Here's how the part is built. I have some questions about the finished solid (model axes, mm). Face numbers are marked on the shaded views. A direction names the side the tool comes from. Coordinates: 2 decimals unless noted, no trailing zeros. Loops run counter-clockwise (first coordinate to the right, second up) from the corner with the lowest first, then second, coordinate; pieces in that order, holes last. Notation, with made-up numbers: M 23.25,-1 L 33.25,-1 A29 ccw 33.25,30 Z; hole C 75.5,-5.75 d1. An arc over 180 degrees is marked long. Use one line per item in the form item = value. Start each with the question number.
(1) Imagine slicing it at C-C, the plane y = 4.75. Please give me the cut outline in (x, z).
(2) Imagine slicing it at D-D, the plane z = 0. Please give me the cut outline in (x, y).
(3) Imagine slicing it at B-B, the plane z = 7.25. Please give me the cut outline in (x, y), and give its area (3 significant figures).
(4) On a 3-axis mill with a long thin cutter (end or side, diameter ignored), from which of +Z, -Z, +X, -X, +Y, -Y can I reach the whole of each face in a straight line? I mean the marked faces 5, 6, 7 and 8. Say none if no direction works.
(5) Please list where these lines run through material, in increasing order: L1, parallel to Z at x = 11.5, y = 3.25; L2, parallel to Z at x = 0, y = 7; L3, parallel to X at y = 6.5, z = 0.
(6) Thinking about a two-plate mould opening in X: for the marked faces 1, 2, 3 and 4, which applies, +X half, -X half, draft (parallel to the pull), parting line (faces both ways), or undercut?
(7) Will these pins go through, and if not, where does the flat tip stop? P1, Ø5, axis at x = 21, y = 5, coming from the -Z side; P2, Ø12, axis at x = -0.5, z = 2.5, coming from the +Y side; P3, Ø1, axis at x = 16, y = 1.5, coming from the +Z side.
(8) Imagine slicing it at A-A, the plane x = 32. Please give me the cut outline in (y, z), and give its area (3 significant figures).
```python
from build123d import *

# Parameters (mm, degrees)
EXTRUDE_1_DEPTH     = 10
SKETCH_2_W          = 5
SKETCH_2_H          = 10
CUT_EXTRUDE_1_DEPTH = 10


with BuildPart() as part:
    # 草图1 → 凸台-拉伸1 (new body)
    with BuildSketch(Plane(origin=(0, 0, 0), x_dir=(1, 0, 0), z_dir=(0, 1, 0))):
        with BuildLine():
            ThreePointArc((11.180339887, 10), (12.90569415, 7.644805982), (14.142135624, 5))
            Line((14.142135624, 5), (50, 5))
            Line((50, 5), (55, 5))
            Line((55, 5), (55, 10))
            Line((55, 10), (11.180339887, 10))
        make_face()
        with BuildLine():
            Line((8.947765084, 5), (14.142135624, 5))
            ThreePointArc((14.142135624, 5), (12.90569415, 7.644805982), (11.180339887, 10))
            ThreePointArc((11.180339887, 10), (-15, 0), (11.180339887, -10))
            ThreePointArc((11.180339887, -10), (12.90569415, -7.644805982), (14.142135624, -5))
            Line((14.142135624, -5), (8.947765084, -5))
            ThreePointArc((8.947765084, -5), (-10.25, 0), (8.947765084, 5))
        make_face()
        with BuildLine():
            Line((50, -5), (14.142135624, -5))
            ThreePointArc((14.142135624, -5), (12.90569415, -7.644805982), (11.180339887, -10))
            Line((11.180339887, -10), (55, -10))
            Line((55, -10), (55, -5))
            Line((55, -5), (50, -5))
        make_face()
    extrude(amount=EXTRUDE_1_DEPTH)

    # 草图2 → 切除-拉伸1 (cut)
    with BuildSketch(Plane(origin=(55, 0, 0), x_dir=(0, 0, -1), z_dir=(1, 0, 0))):
        with Locations((7.5, 5)):
            Rectangle(SKETCH_2_W, SKETCH_2_H)
        with Locations((-7.5, 5)):
            Rectangle(SKETCH_2_W, SKETCH_2_H)
    extrude(amount=-CUT_EXTRUDE_1_DEPTH, mode=Mode.SUBTRACT)


solid = part.part
```
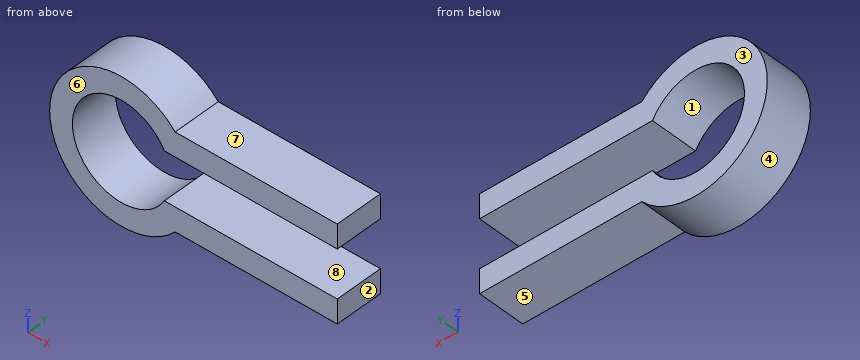
Answer:
q1.outline = M 8.95,-5 A10.25 cw long 8.95,5 L 45,5 L 45,10 L 11.18,10 A15 ccw long 11.18,-10 L 45,-10 L 45,-5 Z
q2.outline = M -15,0 L -10.25,0 L -10.25,10 L -15,10 Z
q3.outline = M -13.13,0 L -7.25,0 L -7.25,10 L -13.13,10 Z; M 7.25,0 L 45,0 L 45,10 L 7.25,10 Z
q3.area = 436 mm²
q4.face_5 = -Z, +X, +Y, -Y
q4.face_6 = +Z, -Z, +X, -X, -Y
q4.face_7 = +Z, +X, +Y, -Y
q4.face_8 = +X, +Y, -Y
q5.L1 = -10 to -5, 5 to 10
q5.L2 = -15 to -10.25, 10.25 to 15
q5.L3 = -15 to -10.25
q6.face_1 = undercut
q6.face_2 = +X half
q6.face_3 = draft
q6.face_4 = parting line
q7.P1 = -10
q7.P2 = through
q7.P3 = 10
q8.outline = M 0,-10 L 10,-10 L 10,-5 L 0,-5 Z; M 0,5 L 10,5 L 10,10 L 0,10 Z
q8.area = 100 mm²
